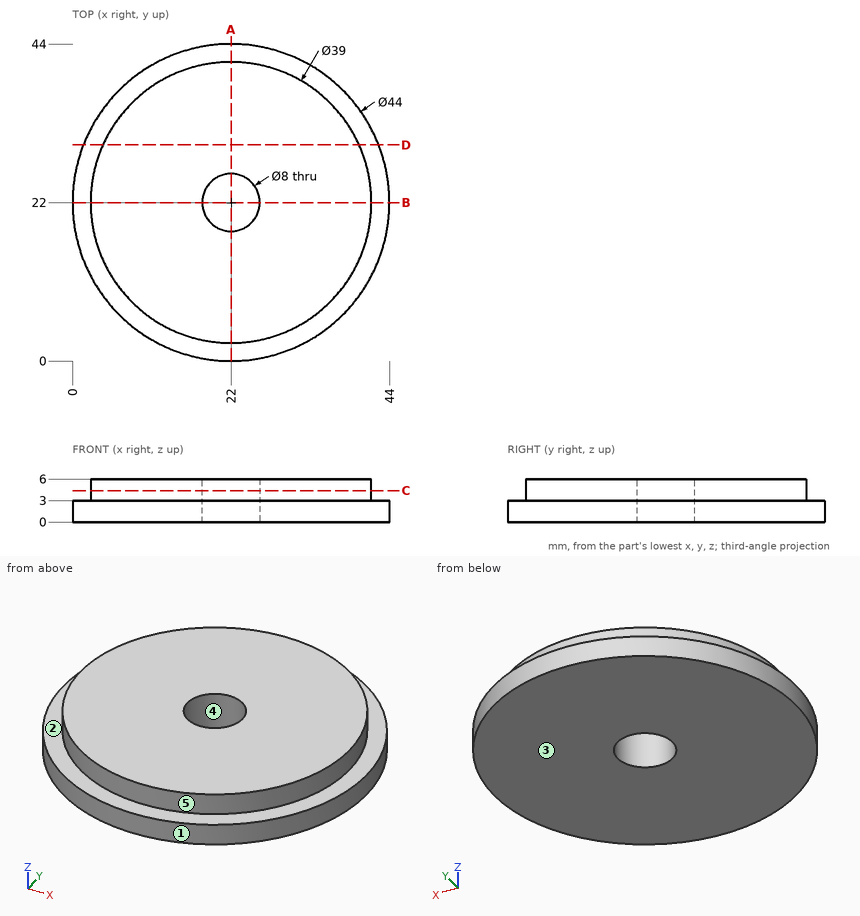
Check sheet for the drawn part. Datum: minimum x, y, z corner. Units: mm. A direction names the side the tool comes from. Round coordinates to 2 decimals unless told otherwise and drop trailing zeros. Loops run counter-clockwise (first coordinate to the right, second up) from the corner with the lowest first, then second, coordinate; pieces in that order, holes last. Notation, with made-up numbers: (-20, 12) - (31, 12) arc R18 ccw to (31, 27) - close; hole circle Ø9 at (78.5, 14.25). An arc over 180 degrees is marked (long way). Write item = value, one per line. Start each with the question number.
1. Mould release check, pull along X, two halves, no side actions. Record for the marked faces 3, 4 and 5: released by +X, released by -X, zero draft, split by the parting line, or undercut.
2. Thickness scan on line 1 (Y direction, x = 22, z = 2.75); line 2 (Y direction, x = 22, z = 4.35); line 3 (Z direction, x = 2, y = 16.5). Record the ranges inside material, lowest first.
3. Set-up check for the marked faces 1 and 2: record each of +Z, -Z, +X, -X, +Y, -Y from which the full face is reachable in a straight line by a thin tool's end or side.
4. Section check D-D on y = 30. Enter the section's corners in (x, z).
5. Depth check by flat-ended pin: pin 1 (2 mm diameter, centred on x = 10.5, z = 3, fed in from -Y); pin 2 (2 mm diameter, centred on x = 6.5, z = 2, fed in from +Y); pin 3 (1.5 mm diameter, centred on x = 31, z = 1, fed in from -Y); pin 4 (6.5 mm diameter, centred on x = 22, y = 22, fed in from -Z). Enter the tip coordinate at first touch or a pass-through.
6. Section check A-A on x = 22. Enter the section's corners in (y, z).
7. Section check C-C on z = 4.4. Enter the section's corners in (x, y).
Working result:
q1.face_3 = zero draft
q1.face_4 = undercut
q1.face_5 = split by the parting line
q2.line_1 = 0 to 18, 26 to 44
q2.line_2 = 2.5 to 18, 26 to 41.5
q2.line_3 = 0 to 3
q3.face_1 = +Z, -Z
q3.face_2 = +Z
q4.outline = (1.51, 0) - (42.49, 0) - (42.49, 3) - (39.78, 3) - (39.78, 6) - (4.22, 6) - (4.22, 3) - (1.51, 3) - close
q5.pin_1 = 2.67
q5.pin_2 = 38.55
q5.pin_3 = 1.61
q5.pin_4 = through
q6.outline = (0, 0) - (18, 0) - (18, 6) - (2.5, 6) - (2.5, 3) - (0, 3) - close; (26, 0) - (44, 0) - (44, 3) - (41.5, 3) - (41.5, 6) - (26, 6) - close
q7.outline = circle Ø39 at (22, 22); hole circle Ø8 at (22, 22)
